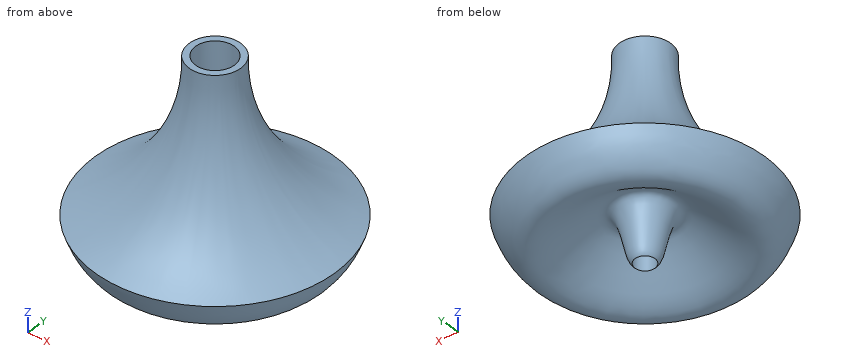
from build123d import *

# Parameters (mm, degrees)
F2_R     = 4.953
F3_DEPTH = 9.525
F4_DEPTH = 17.78


with BuildPart() as f1:
    # F0 (on Front) → F1 (revolve)
    with BuildSketch(Plane.XZ):
        with BuildLine():
            Line((0, 50.8), (0, 0))
            Line((0, 0), (2.54, 0))
            add(Edge.make_bspline(
                [(2.54, 0), (4.6722859433, 1.6956295225), (4.2763701134, 21.355319139), (23.4021219766, -4.0701360184), (29.4854754081, 8.3711690183), (30.601150829, 11.8996728591)],
                knots=[0, 0, 0, 0, 0.3185237965, 0.6935888291, 1, 1, 1, 1], degree=3))
            ThreePointArc((30.601150829, 11.8996728591), (12.7701470866, 27.7559149939), (6.5786, 50.8))
            Line((6.5786, 50.8), (0, 50.8))
        make_face()
    revolve(axis=Axis((0, 0, 25.4), (0, 0, 1)))

    # F2 (on face) → F3 (cut)
    with BuildSketch(Plane.XY.offset(50.8)):
        Circle(F2_R)
    extrude(amount=-F3_DEPTH, mode=Mode.SUBTRACT)

    # F4 (cut): a face of the model
    f4_faces = [f1.faces().sort_by_distance(p)[0] for p in [
        (0, 0, 0),
    ]]
    extrude(f4_faces, amount=-F4_DEPTH, mode=Mode.SUBTRACT)


solid = f1.part
CAD build for the part. Positions are in the model's coordinates, mm. Coordinates: 2 decimals unless noted, no trailing zeros. Write each loop counter-clockwise with the first axis right and the second up, starting at its lowest first coordinate (ties: lowest second). Pieces come first, ordered by that corner, then holes. Notation, with made-up numbers: M -19.5,25.5 L -11.5,25.5 A31 ccw -11.5,57.5 Z; hole C 87.5,-31 d1. An arc over 180 degrees is marked long. Return JSON: item names as keys, results as strings.
Item 1: Slice it at C-C, the plane z = 11. State how many separate pieces and enclosed holes the cut face has, and give its area (3 significant figures).
Findings below:
{"separate pieces": "2", "enclosed holes": "2", "area": "2,640 mm2"}
Item 2: Probe line 1 (X direction, y = 4, z = 8); line 2 (Y direction, x = 0, z = 7); line 3 (Y direction, x = 0, z = 6.5). List the from-to ranges inside material, lowest first. Write a range as from..to.
Findings below:
{"line 1": "x = -28.69..-13.94, -3.13..3.13, 13.94..28.69", "line 2": "y = -28.38..-15.75, -4.84..-2.54, 2.54..4.84, 15.75..28.38", "line 3": "y = -28.05..-16.39, -4.73..-2.54, 2.54..4.73, 16.39..28.05"}
Item 3: Drop flat-ended pins along their axis: pin 1 Ø1.5 at (x, y) = (6.5, -24) entering from -Z; pin 2 Ø3 at (y, z) = (-2.5, 37.5) entering from -X; pin 3 Ø4.5 at (x, y) = (0, 0) entering from +Z (3 decimals). Give the stop position or say it passes through.
Findings below:
{"pin 1": "stops at z = 3.31", "pin 2": "stops at x = -8.61", "pin 3": "stops at z = 41.275"}
Item 4: Slice it at B-B, the plane z = 35.5. Write the cut outline in (x, y), and give its area (3 significant figures).
Findings below:
{"outline": "C 0,0 d18.06", "area": "256 mm2"}
Item 5: Slice it at A-A, the plane z = 43.5. Write the cut outline in (x, y).
Findings below:
{"outline": "C 0,0 d14.03; hole C 0,0 d9.91"}
